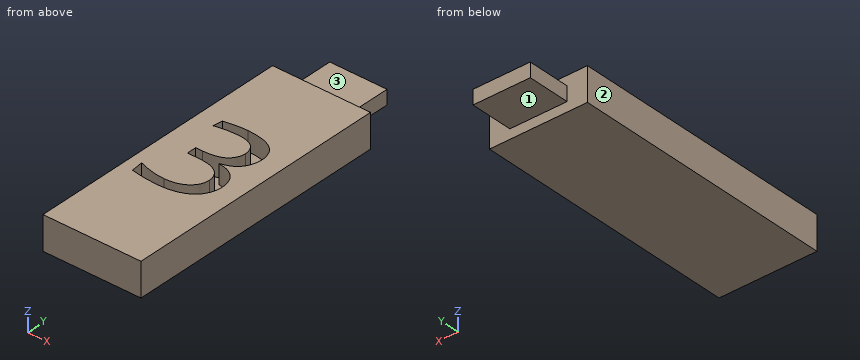
```python
from build123d import *

# Parameters (mm, degrees)
SKETCH1_W           = 17.38
SKETCH1_H           = 47.498
BOSS_EXTRUDE1_DEPTH = 5.95
CUT_EXTRUDE1_DEPTH  = 3.41
SKETCH3_W           = 10.16
SKETCH3_H           = 2.54
BOSS_EXTRUDE2_DEPTH = 7.62


with BuildPart() as part:
    # Sketch1 → Boss-Extrude1 (new body)
    with BuildSketch(Plane.XY):
        Rectangle(SKETCH1_W, SKETCH1_H)
    extrude(amount=BOSS_EXTRUDE1_DEPTH)

    # Sketch2 → Cut-Extrude1 (cut)
    with BuildSketch(Plane.XY.offset(5.95)):
        with BuildLine():
            add(Edge.make_bspline(
                [(-6.52556172, -7.745867902), (-6.541736639, -7.548099343), (-6.573175083, -7.163705708), (-6.622418565, -6.602266915), (-6.692949133, -6.075060478), (-6.743124974, -5.734210105), (-6.767407423, -5.569256574)],
                knots=[0, 0, 0, 0, 1.086986854, 2.112726256, 3.08665945, 4, 4, 4, 4], degree=3))
            add(Edge.make_bspline(
                [(-6.767407423, -5.569256574), (-6.530107504, -5.65714284), (-6.071226782, -5.827093648), (-5.393252267, -6.037243911), (-4.756216501, -6.210347647), (-4.152431156, -6.334769991), (-3.57872429, -6.427846187), (-3.025776205, -6.484148091), (-2.49184335, -6.53213088), (-2.140956001, -6.53515245), (-1.968281752, -6.536639386)],
                knots=[0, 0, 0, 0, 1.233271994, 2.384850126, 3.458654952, 4.449698821, 5.388467082, 6.290264974, 7.158626795, 8, 8, 8, 8], degree=3))
            add(Edge.make_bspline(
                [(-1.968281752, -6.536639386), (-1.75133924, -6.531980014), (-1.327278106, -6.522872262), (-0.706888473, -6.439166817), (-0.115695472, -6.315014093), (0.441587435, -6.128655567), (0.959134586, -5.891680706), (1.434346256, -5.60536251), (1.852688666, -5.254947102), (2.223631893, -4.861847073), (2.530540018, -4.420139374), (2.745748542, -3.932531949), (2.886322279, -3.410547349), (2.899628723, -3.048438292), (2.906420702, -2.86360777)],
                knots=[0, 0, 0, 0, 1.146655432, 2.241386427, 3.304909894, 4.337056057, 5.341489706, 6.310260062, 7.261210465, 8.21792905, 9.162042711, 10.089298595, 11.024724922, 12, 12, 12, 12], degree=3))
            add(Edge.make_bspline(
                [(2.906420702, -2.86360777), (2.901024718, -2.714484768), (2.890393101, -2.420670199), (2.793891256, -1.993867016), (2.631400278, -1.594911679), (2.411871676, -1.222767409), (2.129631062, -0.880783066), (1.777265044, -0.58591917), (1.362310422, -0.334947261), (0.882019785, -0.126391182), (0.326060942, 0.041506515), (-0.317039003, 0.152592763), (-1.047099623, 0.225103406), (-1.563744548, 0.231610819), (-1.836022383, 0.235040301)],
                knots=[0, 0, 0, 0, 0.838837545, 1.652747662, 2.448248001, 3.255922832, 4.076848485, 4.9323124, 5.830012564, 6.798601416, 7.873321705, 9.091954711, 10.467426588, 12, 12, 12, 12], degree=3))
            add(Edge.make_bspline(
                [(-1.836022383, 0.235040301), (-2.118175703, 0.235040301), (-2.71397267, 0.235040301), (-3.309769636, 0.235040301), (-3.623413283, 0.235040301)],
                knots=[0, 0, 0, 0, 0.947145877, 2, 2, 2, 2], degree=3))
            add(Edge.make_bspline(
                [(-3.623413283, 0.235040301), (-3.623413283, 0.401309222), (-3.623413283, 0.716212481), (-3.623413283, 1.164634723), (-3.623413283, 1.562672442), (-3.623413283, 1.812075824), (-3.623413283, 1.927960223)],
                knots=[0, 0, 0, 0, 1.178571429, 2.232142857, 3.178571429, 4, 4, 4, 4], degree=3))
            add(Edge.make_bspline(
                [(-3.623413283, 1.927960223), (-3.414317518, 1.927960223), (-3.017539412, 1.927960223), (-2.620761305, 1.927960223), (-2.433078962, 1.927960223)],
                knots=[0, 0, 0, 0, 1.053968254, 2, 2, 2, 2], degree=3))
            add(Edge.make_bspline(
                [(-2.433078962, 1.927960223), (-2.213703602, 1.930624231), (-1.782777551, 1.935857226), (-1.151023939, 2.0055806), (-0.542619853, 2.10015175), (0.035880784, 2.240575523), (0.575646904, 2.432273783), (1.055902319, 2.692411738), (1.469541725, 3.020520175), (1.811722492, 3.405969987), (2.08288473, 3.830741215), (2.27766536, 4.278496537), (2.402253448, 4.741516196), (2.415895086, 5.057332232), (2.422729296, 5.21555025)],
                knots=[0, 0, 0, 0, 1.198563504, 2.354376706, 3.470500059, 4.562664134, 5.603894105, 6.593029745, 7.533946595, 8.475140529, 9.397714259, 10.276520456, 11.136568486, 12, 12, 12, 12], degree=3))
            add(Edge.make_bspline(
                [(2.422729296, 5.21555025), (2.41848686, 5.321507932), (2.410108472, 5.530763797), (2.361808308, 5.839798802), (2.272318537, 6.136976064), (2.152371646, 6.424223648), (1.999138717, 6.693438231), (1.814730838, 6.941867492), (1.595760775, 7.159214462), (1.345598912, 7.350011462), (1.071173531, 7.516024108), (0.768770465, 7.652369954), (0.443224079, 7.761631168), (-0.02126237, 7.869550376), (-0.625047542, 7.953947292), (-1.113972164, 7.967357708), (-1.359888655, 7.974102801)],
                knots=[0, 0, 0, 0, 0.840069058, 1.659052692, 2.470886163, 3.294117981, 4.121275006, 4.91992718, 5.738789114, 6.557468464, 7.408382134, 8.275078447, 9.181128571, 10.125473558, 12.051213004, 14, 14, 14, 14], degree=3))
            add(Edge.make_bspline(
                [(-1.359888655, 7.974102801), (-1.673695553, 7.969028927), (-2.28838471, 7.959090155), (-3.055728965, 7.892689053), (-3.677904349, 7.813221258), (-4.183457732, 7.722552933), (-4.735878517, 7.618644903), (-5.117536064, 7.534329474), (-5.316333204, 7.490411395)],
                knots=[0, 0, 0, 0, 1.413699745, 2.769173996, 3.467485544, 4.239092287, 5.082781358, 6, 6, 6, 6], degree=3))
            add(Edge.make_bspline(
                [(-5.316333204, 7.490411395), (-5.295473469, 7.596092866), (-5.249427147, 7.829376891), (-5.190410995, 8.217774099), (-5.130669891, 8.676445311), (-5.094041399, 9.006913098), (-5.074487501, 9.183331317)],
                knots=[0, 0, 0, 0, 0.755535026, 1.667787633, 2.754962612, 4, 4, 4, 4], degree=3))
            add(Edge.make_bspline(
                [(-5.074487501, 9.183331317), (-4.839061429, 9.226846422), (-4.393892492, 9.309129464), (-3.762770018, 9.415006617), (-3.207342126, 9.499542218), (-2.574147348, 9.578446025), (-1.850277468, 9.651295087), (-1.284507474, 9.661865299), (-1.008456617, 9.667022723)],
                knots=[0, 0, 0, 0, 1.050947891, 1.987245303, 2.809118091, 3.516901663, 4.788445072, 6, 6, 6, 6], degree=3))
            add(Edge.make_bspline(
                [(-1.008456617, 9.667022723), (-0.787984528, 9.663669776), (-0.351690808, 9.657034605), (0.292002393, 9.617988713), (0.915587457, 9.538862965), (1.515964453, 9.441265363), (2.084281473, 9.307972062), (2.610568352, 9.135217425), (3.086978216, 8.919091142), (3.518718882, 8.670307938), (3.898229552, 8.382060206), (4.228524929, 8.059813131), (4.498719018, 7.696298707), (4.713843094, 7.300619566), (4.879671631, 6.881272468), (4.99630019, 6.442360068), (5.071173168, 5.989007724), (5.079061327, 5.680639804), (5.08303203, 5.525415057)],
                knots=[0, 0, 0, 0, 1.266958933, 2.507193661, 3.702999241, 4.87743226, 6.000982662, 7.053838483, 8.05478712, 9.001953689, 9.911049213, 10.786233696, 11.644646876, 12.503029542, 13.3672512, 14.229318255, 15.108682819, 16, 16, 16, 16], degree=3))
            add(Edge.make_bspline(
                [(5.08303203, 5.525415057), (5.073346612, 5.29136261), (5.053796783, 4.818932278), (4.907815231, 4.243673456), (4.760384651, 3.797657776), (4.628071558, 3.484699001), (4.479730584, 3.193737158), (4.263994326, 2.846554659), (3.965197708, 2.465414494), (3.563814241, 2.084654396), (3.127194483, 1.784257241), (2.736903149, 1.573559514), (2.382780475, 1.423099561), (2.056319362, 1.304292136), (1.671494725, 1.171074546), (1.392673252, 1.085594852), (1.243731493, 1.039933032)],
                knots=[0, 0, 0, 0, 1.526412492, 3.08103406, 3.853748594, 4.594850058, 5.297651013, 5.984869021, 7.262097787, 8.449404989, 9.583765836, 10.713822146, 11.340398739, 12.095345308, 12.982565373, 14, 14, 14, 14], degree=3))
            add(Edge.make_bspline(
                [(1.243731493, 1.039933032), (1.403759525, 1.020356376), (1.704175687, 0.983605665), (2.122673042, 0.923789077), (2.475141845, 0.846858293), (2.864130218, 0.743713734), (3.303014609, 0.555758637), (3.794772208, 0.258479198), (4.254320263, -0.114504015), (4.574491765, -0.49806429), (4.798045633, -0.832017921), (4.936330324, -1.107824276), (5.058160875, -1.397737762), (5.187274335, -1.807722085), (5.303551629, -2.343509578), (5.317731548, -2.782293192), (5.324877733, -3.003424817)],
                knots=[0, 0, 0, 0, 1.05140306, 1.973769637, 2.755120881, 3.402765032, 4.595667385, 5.852196341, 7.141559267, 8.435179725, 9.093568746, 9.758483696, 10.443391522, 11.14214712, 12.559741904, 14, 14, 14, 14], degree=3))
            add(Edge.make_bspline(
                [(5.324877733, -3.003424817), (5.318853578, -3.20043409), (5.306908792, -3.591067038), (5.195219007, -4.166898163), (5.021598461, -4.725154765), (4.780241026, -5.261346273), (4.473837665, -5.76351089), (4.109742558, -6.225711012), (3.681374753, -6.635564365), (3.200544791, -6.997013579), (2.674933003, -7.311812541), (2.107945699, -7.568355733), (1.514168959, -7.792857134), (0.885662086, -7.953548794), (0.235517943, -8.078548986), (-0.432333007, -8.163130761), (-1.114600952, -8.218254877), (-1.57391487, -8.225766961), (-1.80579167, -8.229559308)],
                knots=[0, 0, 0, 0, 0.951341382, 1.886333989, 2.824097537, 3.772375449, 4.720457901, 5.660826572, 6.608087648, 7.57733893, 8.562991247, 9.562683413, 10.581673707, 11.627217792, 12.693490673, 13.78016521, 14.879354254, 16, 16, 16, 16], degree=3))
            add(Edge.make_bspline(
                [(-1.80579167, -8.229559308), (-2.149802637, -8.224115148), (-2.847428076, -8.213074847), (-3.73293587, -8.146076159), (-4.482524718, -8.068898196), (-5.10897433, -7.976987959), (-5.797472847, -7.874373492), (-6.276345169, -7.789853906), (-6.52556172, -7.745867902)],
                knots=[0, 0, 0, 0, 1.303243722, 2.642869155, 3.362762632, 4.157791809, 5.041271022, 6, 6, 6, 6], degree=3))
        make_face()
    extrude(amount=-CUT_EXTRUDE1_DEPTH, mode=Mode.SUBTRACT)

    # Sketch3 → Boss-Extrude2 (add)
    with BuildSketch(Plane(origin=(0, 23.749, 0), x_dir=(1, 0, 0), z_dir=(0, 1, 0))):
        with Locations((0, -2.975)):
            Rectangle(SKETCH3_W, SKETCH3_H)
    extrude(amount=BOSS_EXTRUDE2_DEPTH)


solid = part.part
```
Geometry check sheet. Reference: the model listing, model coordinates, mm. Face numbers are marked on the shaded views. A direction names the side the tool comes from. Round coordinates to 2 decimals unless told otherwise and drop trailing zeros. Order: outer loops, then holes, each group sorted by start corner. A loop starts at its lowest first (then second) coordinate and runs counter-clockwise, first axis right, second up. Notation, with made-up numbers: (39, 89.25) - (75, 89.25) arc R17 ccw to (75, 111.25) - close; hole circle Ø11 at (15, 4). An arc over 180 degrees is marked (long way). Use a Markdown table: item, result. Add a question column.
1) Set-up check for the marked faces 1, 2 and 3: record each of +Z, -Z, +X, -X, +Y, -Y from which the full face is reachable in a straight line by a thin tool's end or side.
2) Section check B-B (y = 26.5). Record the cut outline in (x, z) (3 decimals), then the cut area to 3 significant figures.
3) Gauge pin test, flat ends, axial feed: P1, Ø2, axis at y = 29, z = 2.5, coming from the -X side; P2, Ø2, axis at x = 2, z = 1.5, coming from the +Y side; P3, Ø2.5, axis at x = -0.5, y = 28.5, coming from the +Z side (3 decimals); P4, Ø0.8, axis at y = 27.5, z = 3, coming from the +X side. Record the tip position at first contact, or that the pin passes through.
4) Thickness scan on line 1 along Y through (x, z) = (-3, 5.7) (3 decimals); line 2 along Y through (x, z) = (0.5, 3.35); line 3 along Y through (x, z) = (2, 5). Record the ranges inside material, lowest first.
5) Section check A-A (x = -7.25). Record the cut outline in (y, z), then the cut area to 3 significant figures.
Established:
| question | item | result |
|---|---|---|
| 1 | face 1 | -Z, +X, -X, +Y |
| 1 | face 2 | +Z, -Z, -X, +Y, -Y |
| 1 | face 3 | +Z, +X, -X, +Y |
| 2 | outline | (-5.08, 1.705) - (5.08, 1.705) - (5.08, 4.245) - (-5.08, 4.245) - close |
| 2 | area | 25.8 mm2 |
| 3 | P1 | x = -5.08 |
| 3 | P2 | y = 31.37 |
| 3 | P3 | z = 4.245 |
| 3 | P4 | x = 5.08 |
| 4 | line 1 | -23.749 to -8.195, -6.486 to 0.235, 1.928 to 7.894, 9.525 to 23.749 |
| 4 | line 2 | -23.75 to -8.03, -6.09 to -0.02, 2.42 to 7.74, 9.59 to 31.37 |
| 4 | line 3 | -23.75 to -7.61, -5.09 to -0.78, 0.94 to 1.29, 3.71 to 6.68, 9.32 to 23.75 |
| 5 | outline | (-23.75, 0) - (23.75, 0) - (23.75, 5.95) - (-23.75, 5.95) - close |
| 5 | area | 283 mm2 |
